Could you check a few things on this model? Use its own coordinates, in mm. A direction names the side the tool comes from. Give positions to 0.01 mm unless a question says otherwise; leave off trailing zeros. Loops run counter-clockwise (first coordinate to the right, second up) from the corner with the lowest first, then second, coordinate; pieces in that order, holes last. Notation, with made-up numbers: (0, 18.5) -> (34, 18.5) arc R7 ccw to (34, 22.5) -> close; hole circle Ø1 at (62, 8.25). An arc over 180 degrees is marked (long way). Write item = value, one per line. Start each with the question number.
1) I want a section at A-A (z = 0). Count the separate pieces of the cut face and the enclosed holes in it, and give its area (3 significant figures).
2) On a 3-axis mill with a long thin cutter (end or side, diameter ignored), from which of +Z, -Z, +X, -X, +Y, -Y can I reach the whole of each face in a straight line? I mean faces 4 (the face through (0.27, -6.01, -33.78)), 5 (the face through (32.35, -2, 0)), 6 (the face through (-8.67, -3.45, 39.05)). Say none if no direction works.
3) I want a section at C-C (y = 28.5). List the corners of the cut face in (x, z) for me, and give its area (3 significant figures).
4) I need wall thicknesses on probe 1 along Z at (x, y) = (0, -4.7); probe 2 along Z at (x, y) = (0, -5.4); probe 3 along Y at (x, z) = (25, -28). Which ranges of each line are inside material? Lowest first, please. Write a range as from..to.
5) If we mould it in two halves opening along Z, with no side actions, what happens to faces 1 (the face through (-34, -5, 1)), 2 (the face through (-2.306, -2.465, 33.694)), 3 (the face through (-8.67, 44.93, -39.05))? For each: +Z half, -Z half, draft (parallel to the pull), parting line (faces both ways), or undercut.
6) I want a section at D-D (y = 36.5). List the corners of the cut face in (x, z) for me, and give its area (3 significant figures).
7) I'm going to push flat-ended pins straight in: pin 1 Ø3 at (y, z) = (29, -14) entering from +X; pin 2 Ø2.5 at (x, y) = (0, -2.5) entering from +Z; pin 3 Ø1.5 at (x, y) = (24.5, 1.5) entering from +Z. Where does each tip first touch, or does it pass through?
Autodesk Inventor part; units mm, degrees
ref_plane "YZ Plane" through (0, 0, 0) normal (1, 0, 0) x (0, 1, 0)
ref_plane "XZ Plane" through (0, 0, 0) normal (0, 1, 0) x (-1, 0, 0)
ref_plane "XY Plane" through (0, 0, 0) normal (0, 0, 1) x (1, 0, 0)
sketch "Sketch1" plane through (0, 0, 0) normal (0, 1, 0) x (-1, 0, 0)
  circle A0 centre (0, 0) radius 30
  circle A1 centre (0, 0) radius 45
  circle A2 centre (0, 0) radius 20
  dimension "d0" = 60
  dimension "d1" = 90
  dimension "d2" = 40
extrude "Extrusion1" add sketch "Sketch1" along normal blind 20 draft -4 contours A0
sketch "Sketch2" plane through (0, 20, 0) normal (0, 1, 0) x (1, 0, 0)
  circle A0 centre (0, 0) radius 28.6015
  circle A1 centre (0, 0) radius 21.3985
extrude "Extrusion2" add sketch "Sketch2" along normal blind 20 draft 4
sketch "Sketch3" plane through (0, 40, 0) normal (0, 1, 0) x (1, 0, 0)
  circle A0 centre (0, 0) radius 40
  dimension "d7" = 80
extrude "Extrusion3" add sketch "Sketch3" along normal blind 10
sketch "Sketch4" plane through (0, 0, 0) normal (0, -1, 0) x (1, 0, 0)
  circle A0 centre (0, 0) radius 40
  dimension "d10" = 80
extrude "Extrusion4" add sketch "Sketch4" along normal blind 10
ref_plane "Work Plane1" through (0, -8, 0) normal (0, -1, 0) x (1, 0, 0)
sketch "Sketch7" plane through (0, -10, 0) normal (0, -1, 0) x (1, 0, 0)
  circle A0 centre (0, 0) radius 40
extrude "Extrusion12" cut sketch "Sketch7" against normal blind 3
sketch "Sketch8" plane through (0, -7, 0) normal (0, -1, 0) x (1, 0, 0)
  circle A0 centre (0, 0) radius 25
  dimension "d42" = 50
extrude "Extrusion13" cut sketch "Sketch8" against normal blind 5
sketch "Sketch9" plane through (0, 0, 0) normal (0, 1, 0) x (1, 0, 0)
  circle A0 centre (0, 0) radius 35
  line L0 (-37.65, 1.53) -> (-35, 3.06)
  line L1 (-35, 3.06) -> (-32.35, 1.53)
  line L2 (-32.35, 1.53) -> (-32.35, -1.53)
  line L3 (-32.35, -1.53) -> (-35, -3.06)
  line L4 (-35, -3.06) -> (-37.65, -1.53)
  line L5 (-37.65, -1.53) -> (-37.65, 1.53)
  line L6 (0, 0) -> (-35, 0) construction
  circle A1 centre (-35, 0) radius 2.65
  point P0 (-33.675, 2.295)
  point P1 (-36.325, -2.295)
  dimension "d45" = 70
  dimension "d46" = 5.3
extrude "Extrusion14" cut sketch "Sketch9" against normal through all contours L1 A1 A0 | A0 A1 L0 L1 | L3 L4 A1 A0 | A0 A1 L3 | A1 A0 | A0 A1 | L1 L2 A1 | A1 L2 L3 | A1 L5 L0 | L4 L5 A1
pattern_circular "Circular Pattern1" count 4 over 360 about axis through (0, 0, 0) along (0, -1, 0) of "Extrusion14"
sketch "Sketch10" plane through (0, 0, 0) normal (0, 0, 1) x (1, 0, 0)
  point P0 (0, 0)
sketch "Sketch11" plane through (0, 0, 0) normal (0, 0, 1) x (1, 0, 0)
  line L0 (-24.5677, 41.8645) -> (0, 41.8645)
  line L1 (0, 41.8645) -> (0, 0)
  line L2 (0, 0) -> (-24.5677, 0)
  line L3 (-24.5677, 0) -> (-24.5677, 41.8645)
revolve "Revolution1" add sketch "Sketch11" angle 360 about axis through (0, 41.8645, 0) along (0, -1, 0)
sketch "Sketch12" plane through (0, -7, 0) normal (0, -1, 0) x (1, 0, 0)
  point P0 (0, 0)
sketch "Sketch13" plane through (0, -7, 0) normal (0, -1, 0) x (1, 0, 0)
  line L0 (0, 35) -> (0, 0) construction
  circle A0 centre (0, 35) radius 3.15
  circle A1 centre (0, 35) radius 1.25
  dimension "d53" = 35
  dimension "d54" = 6.3
  dimension "d57" = 2.5
extrude "Extrusion15" add sketch "Sketch13" against normal blind 2
pattern_circular "Circular Pattern2" count 4 over 360 about axis through (0, 0, 0) along (0, -1, 0) of "Extrusion15"
properties part number "spool" material "ABS Plastic"
Answer list:
q1.separate_pieces = 3
q1.enclosed_holes = 0
q1.area = 3,390 mm^2
q2.face_4 = -Y
q2.face_5 = none
q2.face_6 = +Y, -Y
q3.outline = circle Ø58.39 at (0, 0)
q3.area = 2,680 mm^2
q4.probe_1 = -40..-37.65, -32.35..-25, 25..32.35, 37.65..40
q4.probe_2 = -40..-36.25, -33.75..-25, 25..33.75, 36.25..40
q4.probe_3 = -7..0, 40..50
q5.face_1 = undercut
q5.face_2 = undercut
q5.face_3 = parting line
q6.outline = circle Ø59.51 at (0, 0)
q6.area = 2,780 mm^2
q7.pin_1 = 26.43
q7.pin_2 = 40
q7.pin_3 = 18.16
